Could you check a few things on this model? Use its own coordinates, in mm. A direction names the side the tool comes from. Give positions to 0.01 mm unless a question says otherwise; leave off trailing zeros. Order: outer loops, then holes, each group sorted by start corner. A loop starts at its lowest first (then second) coordinate and runs counter-clockwise, first axis right, second up. Notation, with made-up numbers: M 11,73.5 L 39,73.5 A8 cw 39,81.5 Z; hole C 39,39.25 d6. An arc over 180 degrees is marked long. Use a Markdown table: item, result. Add a question column.
```python
from build123d import *

# Parameters (mm, degrees)
EXTRUDE_1_DEPTH          = 20
SKETCH_2_W               = 4
SKETCH_2_H               = 38.6
CUT_EXTRUDE_1_DEPTH      = 20
CUT_EXTRUDE_2_DEPTH      = 65.286857133
CUT_EXTRUDE_2_DEPTH_BACK = 65.286857133
SKETCH_3_R               = 1.175
EXTRUDE_2_DEPTH          = 20
CUT_EXTRUDE_3_DEPTH      = 17
SKETCH_7_R               = 1
CUT_EXTRUDE_4_DEPTH      = 4.8
SKETCH_8_W               = 4
SKETCH_8_H               = 20.6
CUT_EXTRUDE_5_DEPTH      = 25.4
EXTRUDE_START            = 10
SKETCH_9_R               = 1.9
SKETCH_9_R_2             = 1
EXTRUDE_3_DEPTH          = 10
CUT_EXTRUDE_6_DEPTH      = 2.5
CUT_EXTRUDE_7_DEPTH      = 2.5
CUT_EXTRUDE_10_DEPTH     = 27
SKETCH_15_R              = 0.95
CUT_EXTRUDE_11_DEPTH     = 50
SKETCH_16_R              = 2.5
CUT_EXTRUDE_12_DEPTH     = 2
CUT_EXTRUDE_START        = -2
SKETCH_17_R              = 2.5
CUT_EXTRUDE_13_DEPTH     = 2
SKETCH_18_W              = 3
SKETCH_18_H              = 38.6
EXTRUDE_4_DEPTH          = 10
SKETCH_19_W              = 11.8
SKETCH_19_H              = 17.6
CUT_EXTRUDE_14_DEPTH     = 0.5
SKETCH_20_R              = 0.95
CUT_EXTRUDE_15_DEPTH     = 10.5
SKETCH_21_W              = 8.8
SKETCH_21_H              = 0.7
CUT_EXTRUDE_16_DEPTH     = 12
SKETCH_23_W              = 2.3
SKETCH_23_H              = 48.6
EXTRUDE_5_DEPTH          = 13
SKETCH_26_R              = 0.95
CUT_EXTRUDE_17_DEPTH     = 10
SKETCH_27_R              = 1.25
CUT_EXTRUDE_18_DEPTH     = 2


with BuildPart() as part:
    # 草图1 → 凸台-拉伸1 (new, symmetric)
    with BuildSketch(Plane.XY):
        Polygon((4, 5), (10.5, 5), (10.5, 8), (14.5, 8), (14.5, 5), (42.8, 5), (42.8, 0), (0, 0), (0, 48.6), (42.8, 48.6), (42.8, 43.6), (14.5, 43.6), (14.5, 40.6), (10.5, 40.6), (10.5, 43.6), (4, 43.6), align=None)
    extrude(amount=EXTRUDE_1_DEPTH, both=True)

    # 草图2 → 切除-拉伸1 (cut)
    with BuildSketch(Plane(origin=(0, 0, -20), x_dir=(-1, 0, 0), z_dir=(0, 0, -1))):
        with Locations((-12.5, 24.3)):
            Rectangle(SKETCH_2_W, SKETCH_2_H)
    extrude(amount=-CUT_EXTRUDE_1_DEPTH, mode=Mode.SUBTRACT)

    # 草图3 → 切除-拉伸2 (cut, two sides: drawn at the far end of the back side and taken through both)
    with BuildSketch(Plane.XZ.offset(-43.6).offset(-CUT_EXTRUDE_2_DEPTH_BACK)):
        with Locations((9.1, -17.5)):
            Circle(SKETCH_3_R)
        with Locations((18.6, -17.5)):
            Circle(SKETCH_3_R)
    extrude(amount=CUT_EXTRUDE_2_DEPTH + CUT_EXTRUDE_2_DEPTH_BACK, mode=Mode.SUBTRACT)

    # 草图4 → 凸台-拉伸2 (add)
    with BuildSketch(Plane.XY.offset(20)):
        Polygon((10.5, 40.6), (10.5, 37.6), (4, 37.6), (4, 11), (10.5, 11), (10.5, 8), (14.5, 8), (14.5, 5), (26.5, 5), (26.5, 43.6), (14.5, 43.6), (14.5, 40.6), align=None)
    extrude(amount=-EXTRUDE_2_DEPTH)

    # 草图6 → 切除-拉伸3 (cut)
    with BuildSketch(Plane(origin=(0, 0, 0), x_dir=(-1, 0, 0), z_dir=(0, 0, -1))):
        Polygon((-26.5, 43.6), (-13.5, 43.6), (-13.5, 34.6), (-4, 34.6), (-4, 14), (-13.5, 14), (-13.5, 5), (-26.5, 5), align=None)
    extrude(amount=-CUT_EXTRUDE_3_DEPTH, mode=Mode.SUBTRACT)

    # 草图7 → 切除-拉伸4 (cut)
    with BuildSketch(Plane(origin=(0, 0, 17), x_dir=(-1, 0, 0), z_dir=(0, 0, -1))):
        with Locations((-21.5, 24.3)):
            Circle(SKETCH_7_R)
        with Locations((-11.5, 24.3)):
            Circle(SKETCH_7_R)
        with Locations((-21.5, 6.7)):
            Circle(SKETCH_7_R)
        with Locations((-21.5, 41.9)):
            Circle(SKETCH_7_R)
    extrude(amount=-CUT_EXTRUDE_4_DEPTH, mode=Mode.SUBTRACT)

    # 草图8 → 切除-拉伸5 (cut)
    with BuildSketch(Plane(origin=(0, 0, -20), x_dir=(-1, 0, 0), z_dir=(0, 0, -1))):
        with Locations((-2, 24.3)):
            Rectangle(SKETCH_8_W, SKETCH_8_H)
    extrude(amount=-CUT_EXTRUDE_5_DEPTH, mode=Mode.SUBTRACT)

    # 草图9 → 凸台-拉伸3 (add)
    # profile 1 of 3: a face of its own
    with BuildSketch(Plane(origin=(0, 0, 17), x_dir=(-1, 0, 0), z_dir=(0, 0, -1)).offset(EXTRUDE_START)):
        with Locations((-21.5, 41.9)):
            Circle(SKETCH_9_R)
        with Locations((-21.5, 41.9)):
            Circle(SKETCH_9_R_2, mode=Mode.SUBTRACT)
    # profile 2 of 3: a face of its own
    with BuildSketch(Plane(origin=(0, 0, 17), x_dir=(-1, 0, 0), z_dir=(0, 0, -1)).offset(EXTRUDE_START)):
        with Locations(Location((-11.5, 24.3, 0), (0, 0, 180))):
            Circle(SKETCH_9_R)
        with Locations((-11.5, 24.3)):
            Circle(SKETCH_9_R_2, mode=Mode.SUBTRACT)
    # profile 3 of 3: a face of its own
    with BuildSketch(Plane(origin=(0, 0, 17), x_dir=(-1, 0, 0), z_dir=(0, 0, -1)).offset(EXTRUDE_START)):
        with Locations((-21.5, 6.7)):
            Circle(SKETCH_9_R)
        with Locations((-21.5, 6.7)):
            Circle(SKETCH_9_R_2, mode=Mode.SUBTRACT)
    extrude(amount=-EXTRUDE_3_DEPTH)

    # 草图10 → 切除-拉伸6 (cut)
    with BuildSketch(Plane(origin=(0, 48.6, 0), x_dir=(1, 0, 0), z_dir=(0, 1, 0))):
        Polygon((11.524871131, 17.5), (10.312435565, 19.6), (10.312435565, 20), (7.887564435, 20), (7.887564435, 19.6), (6.675128869, 17.5), (7.887564435, 15.4), (10.312435565, 15.4), align=None)
        Polygon((21.024871131, 17.5), (19.812435565, 19.6), (19.812435565, 20), (17.387564435, 20), (17.387564435, 19.6), (16.175128869, 17.5), (17.387564435, 15.4), (19.812435565, 15.4), align=None)
    extrude(amount=-CUT_EXTRUDE_6_DEPTH, mode=Mode.SUBTRACT)

    # 草图11 → 切除-拉伸7 (cut)
    with BuildSketch(Plane.XZ):
        Polygon((11.524871131, -17.5), (10.312435565, -15.4), (7.887564435, -15.4), (6.675128869, -17.5), (7.887564435, -19.6), (7.887564435, -20), (10.312435565, -20), (10.312435565, -19.6), align=None)
        Polygon((21.024871131, -17.5), (19.812435565, -15.4), (17.387564435, -15.4), (16.175128869, -17.5), (17.387564435, -19.6), (17.387564435, -20), (19.812435565, -20), (19.812435565, -19.6), align=None)
    extrude(amount=-CUT_EXTRUDE_7_DEPTH, mode=Mode.SUBTRACT)

    # 草图14 → 切除-拉伸10 (cut)
    with BuildSketch(Plane(origin=(0, 0, -20), x_dir=(-1, 0, 0), z_dir=(0, 0, -1))):
        Polygon((-42.8, 4.3), (-12.8, 4.3), (-12.8, 13.3), (-4, 13.3), (-4, 14), (-13.5, 14), (-13.5, 5), (-42.8, 5), align=None)
        Polygon((-4, 35.3), (-12.8, 35.3), (-12.8, 44.3), (-42.8, 44.3), (-42.8, 43.6), (-13.5, 43.6), (-13.5, 34.6), (-4, 34.6), align=None)
    extrude(amount=-CUT_EXTRUDE_10_DEPTH, mode=Mode.SUBTRACT)

    # 草图15 → 切除-拉伸11 (cut)
    with BuildSketch(Plane.XZ):
        with Locations((34.8, -12.122060158)):
            Circle(SKETCH_15_R)
    extrude(amount=-CUT_EXTRUDE_11_DEPTH, mode=Mode.SUBTRACT)

    # 草图16 → 切除-拉伸12 (cut)
    with BuildSketch(Plane.XZ):
        with Locations((34.8, -12.122060158)):
            Circle(SKETCH_16_R)
    extrude(amount=-CUT_EXTRUDE_12_DEPTH, mode=Mode.SUBTRACT)

    # 草图17 → 切除-拉伸13 (cut)
    with BuildSketch(Plane(origin=(0, 48.6, 0), x_dir=(1, 0, 0), z_dir=(0, 1, 0)).offset(CUT_EXTRUDE_START)):
        with Locations((34.8, 12.122060158)):
            Circle(SKETCH_17_R)
    extrude(amount=CUT_EXTRUDE_13_DEPTH, mode=Mode.SUBTRACT)

    # 草图18 → 凸台-拉伸4 (add)
    with BuildSketch(Plane(origin=(26.5, 0, 0), x_dir=(0, 0, -1), z_dir=(1, 0, 0))):
        with Locations((-18.5, 24.3)):
            Rectangle(SKETCH_18_W, SKETCH_18_H)
    extrude(amount=EXTRUDE_4_DEPTH)

    # 草图19 → 切除-拉伸14 (cut)
    with BuildSketch(Plane.XY.offset(20)):
        Polygon((15, 48.6), (15.5, 48.6), (15.5, 33.6), (27.3, 33.6), (27.3, 48.6), (27.8, 48.6), (27.8, 33.6), (36.5, 33.6), (36.5, 33.1), (27.8, 33.1), (27.8, 15.5), (36.5, 15.5), (36.5, 15), (27.8, 15), (27.8, 0), (27.3, 0), (27.3, 15), (15.5, 15), (15.5, 0), (15, 0), (15, 15), (0, 15), (0, 15.5), (15, 15.5), (15, 33.1), (0, 33.1), (0, 33.6), (15, 33.6), align=None)
        with Locations((21.4, 24.3)):
            Rectangle(SKETCH_19_W, SKETCH_19_H, mode=Mode.SUBTRACT)
    extrude(amount=-CUT_EXTRUDE_14_DEPTH, mode=Mode.SUBTRACT)

    # 草图20 → 切除-拉伸15 (cut)
    with BuildSketch(Plane(origin=(0, 0, 17), x_dir=(-1, 0, 0), z_dir=(0, 0, -1))):
        with Locations((-31.5, 24.3)):
            Circle(SKETCH_20_R)
    extrude(amount=-CUT_EXTRUDE_15_DEPTH, mode=Mode.SUBTRACT)

    # 草图21 → 切除-拉伸16 (cut)
    with BuildSketch(Plane(origin=(0, 0, -20), x_dir=(-1, 0, 0), z_dir=(0, 0, -1))):
        with Locations((-8.4, 43.95)):
            Rectangle(SKETCH_21_W, SKETCH_21_H)
        with Locations((-8.4, 4.65)):
            Rectangle(SKETCH_21_W, SKETCH_21_H)
    extrude(amount=-CUT_EXTRUDE_16_DEPTH, mode=Mode.SUBTRACT)

    # 草图23 → 凸台-拉伸5 (add)
    with BuildSketch(Plane.XY.offset(20)):
        with Locations((41.65, 24.3)):
            Rectangle(SKETCH_23_W, SKETCH_23_H)
    extrude(amount=-EXTRUDE_5_DEPTH)

    # 草图26 → 切除-拉伸17 (cut)
    with BuildSketch(Plane.XY.offset(20)):
        with Locations((16.9, 9)):
            Circle(SKETCH_26_R)
        with Locations((16.9, 39.6)):
            Circle(SKETCH_26_R)
    extrude(amount=-CUT_EXTRUDE_17_DEPTH, mode=Mode.SUBTRACT)

    # 草图27 → 切除-拉伸18 (cut)
    with BuildSketch(Plane(origin=(0, 0, 7), x_dir=(-1, 0, 0), z_dir=(0, 0, -1))):
        with Locations((-21.5, 41.9)):
            Circle(SKETCH_27_R)
        with Locations((-11.5, 24.3)):
            Circle(SKETCH_27_R)
        with Locations((-21.5, 6.7)):
            Circle(SKETCH_27_R)
    extrude(amount=-CUT_EXTRUDE_18_DEPTH, mode=Mode.SUBTRACT)


solid = part.part
```
1) Suppose I cut it at B-B on y = 20.5. Please give me the cut outline in (x, z), and give its area (3 significant figures).
2) For pin 1 (2.5 mm diameter, centred on x = 34.8, z = -12.12, fed in from -Y); pin 2 (2 mm diameter, centred on x = 23, z = -5.5, fed in from -Y), each with a flat end and sliding along its axis, tell me the tip position at first contact or that it passes through.
3) Suppose I cut it at A-A on z = 10. Please give me the cut outline in (x, y), and give its area (3 significant figures).
4) Suppose I cut it at C-C on z = -6. Please give me the cut outline in (x, y), and give its area (3 significant figures).
5) We'd pull the mould along Y, two halves only. Please class faces 6 (the face through (40.5, 24, 14)), 7 (the face through (7, 24, 20)), 8 (the face through (9, 2.5, -19)): pulls with the +Y half, pulls with the -Y half, needs draft (parallel to the pull), parting line crosses it, or undercut.
6) For faces 1 (the face through (7.29, 47.368, -18.565)), 2 (the face through (10.927, 1.232, -16.465)), 3 (the face through (24, 44.3, -7)), 4 (the face through (13.5, 10, 12)), 5 (the face through (9, 1, -15.4)), which set-ups out of +Z, -Z, +X, -X, +Y, -Y let a thin tool reach every point of the face, with its end or its side?
7) Suppose I cut it at D-D on x = 39. Please give me the cut outline in (y, z).
8) Please list where these lines run through material, in increasing order: line 1 (Z direction, x = 9, y = 45); line 2 (X direction, y = 41, z = 1); line 3 (Y direction, x = 19, z = 10.5). Write a range as from..to.
Values found:
| question | item | result |
|---|---|---|
| 1 | outline | M 0,5.4 L 4,5.4 L 4,17 L 36.5,17 L 36.5,20 L 27.8,20 L 27.8,19.5 L 27.3,19.5 L 27.3,20 L 15.5,20 L 15.5,19.5 L 15,19.5 L 15,20 L 0,20 Z; M 40.5,7 L 42.8,7 L 42.8,20 L 40.5,20 Z |
| 1 | area | 185 mm^2 |
| 2 | pin 1 | stops at y = 2 |
| 2 | pin 2 | stops at y = 0 |
| 3 | outline | M 0,0 L 42.8,0 L 42.8,48.6 L 0,48.6 Z; C 11.5,24.3 d3.8; hole M 4,5 L 10.5,5 L 10.5,11 L 4,11 Z; hole M 4,14 L 13.5,14 L 13.5,5 L 20.65,5 A1.9 cw long 22.35,5 L 40.5,5 L 40.5,43.6 L 22.35,43.6 A1.9 cw long 20.65,43.6 L 13.5,43.6 L 13.5,34.6 L 4,34.6 Z; hole M 4,37.6 L 10.5,37.6 L 10.5,43.6 L 4,43.6 Z; hole C 11.5,24.3 d2; hole C 21.5,6.7 d2; hole C 21.5,41.9 d2 |
| 3 | area | 788 mm^2 |
| 4 | outline | M 0,0 L 42.8,0 L 42.8,4.3 L 12.8,4.3 L 12.8,5 L 4,5 L 4,14 L 0,14 Z; M 0,34.6 L 4,34.6 L 4,43.6 L 12.8,43.6 L 12.8,44.3 L 42.8,44.3 L 42.8,48.6 L 0,48.6 Z |
| 4 | area | 458 mm^2 |
| 5 | face 6 | undercut |
| 5 | face 7 | needs draft |
| 5 | face 8 | pulls with the -Y half |
| 6 | face 1 | +Y |
| 6 | face 2 | -Y |
| 6 | face 3 | -Z, +X |
| 6 | face 4 | -Z |
| 6 | face 5 | -Z, -Y |
| 7 | outline | M 0,-20 L 4.3,-20 L 4.3,7 L 5,7 L 5,20 L 0,20 Z; M 43.6,7 L 44.3,7 L 44.3,-20 L 48.6,-20 L 48.6,20 L 43.6,20 Z |
| 8 | line 1 | z = -20..-18.67, -16.33..20 |
| 8 | line 2 | x = 0..4, 10.5..12.8 |
| 8 | line 3 | y = 0..5, 43.6..48.6 |
